from build123d import *

# Parameters (mm, degrees)
SKETCH1_R           = 2.032
BOSS_EXTRUDE1_DEPTH = 7.62
SKETCH3_W           = 2.54
SKETCH3_H           = 7.62
CUT_EXTRUDE1_DEPTH  = 55.88
FILLET2_R           = 4.064
SKETCH5_W           = 8.89
SKETCH5_H           = 7.62
SKETCH5_R           = 1.905
BOSS_EXTRUDE2_DEPTH = 5.08
FILLET3_R           = 1.27
FILLET4_R           = 0.0508


with BuildPart() as part:
    # Sketch1 → Boss-Extrude1 (new body)
    with BuildSketch(Plane.XY):
        Polygon((0, 0), (0, 12.7), (7.62, 12.7), (7.62, 5.08), (48.26, 5.08), (48.26, 12.7), (55.88, 12.7), (55.88, 0), align=None)
        with Locations((3.81, 8.89)):
            Circle(SKETCH1_R, mode=Mode.SUBTRACT)
        with Locations((52.07, 8.89)):
            Circle(SKETCH1_R, mode=Mode.SUBTRACT)
    extrude(amount=-BOSS_EXTRUDE1_DEPTH)

    # Sketch3 → Cut-Extrude1 (cut)
    with BuildSketch(Plane(origin=(55.88, 0, 0), x_dir=(0, 0, -1), z_dir=(1, 0, 0))):
        with Locations((3.81, 8.89)):
            Rectangle(SKETCH3_W, SKETCH3_H)
    extrude(amount=-CUT_EXTRUDE1_DEPTH, mode=Mode.SUBTRACT)

    # Fillet2
    # the kernel refuses this fillet: 4.064 mm, written as the material it takes off along each edge
    with BuildSketch(Plane(origin=(48.26, 12.7, 5.08), x_dir=(0, -1, 0), z_dir=(0, 0, -1)), Plane(origin=(48.26, 12.7, 10.16), x_dir=(0, -1, 0), z_dir=(0, 0, -1)), Plane(origin=(7.62, 12.7, 5.08), x_dir=(-1, 0, 0), z_dir=(0, 0, -1)), Plane(origin=(7.62, 12.7, 10.16), x_dir=(-1, 0, 0), z_dir=(0, 0, -1)), Plane(origin=(55.88, 12.7, 10.16), x_dir=(-1, 0, 0), z_dir=(0, 0, -1)), Plane(origin=(0, 12.7, 5.08), x_dir=(0, -1, 0), z_dir=(0, 0, -1)), Plane(origin=(0, 12.7, 10.16), x_dir=(0, -1, 0), z_dir=(0, 0, -1))) as fillet2_piece_1:
        with BuildLine():
            CenterArc((FILLET2_R, -FILLET2_R), FILLET2_R, 90, 90)
            Line((0, -FILLET2_R), (0, 0))
            Line((0, 0), (FILLET2_R, 0))
        make_face()
    extrude(amount=22.86, mode=Mode.SUBTRACT)
    with BuildSketch(Plane(origin=(55.88, 12.7, 5.08), x_dir=(0, -1, 0), z_dir=(0, 0, -1))) as fillet2_piece_2:
        with BuildLine():
            CenterArc((FILLET2_R, FILLET2_R), FILLET2_R, 180, 90)
            Line((0, FILLET2_R), (0, 0))
            Line((0, 0), (FILLET2_R, 0))
        make_face()
    extrude(amount=22.86, mode=Mode.SUBTRACT)

    # Sketch5 → Boss-Extrude2 (add)
    # profile 1 of 2: a face of its own
    with BuildSketch(Plane(origin=(0, 0, 0), x_dir=(1, 0, 0), z_dir=(0, 1, 0))):
        with Locations((-4.445, 3.81)):
            Rectangle(SKETCH5_W, SKETCH5_H)
        with Locations(Location((-5.08, 3.81, 0), (0, 0, 270))):
            Circle(SKETCH5_R, mode=Mode.SUBTRACT)
    # profile 2 of 2: a face of its own
    with BuildSketch(Plane(origin=(0, 0, 0), x_dir=(1, 0, 0), z_dir=(0, 1, 0))):
        with Locations((60.325, 3.81)):
            Rectangle(SKETCH5_W, SKETCH5_H)
        with Locations(Location((60.96, 3.81, 0), (0, 0, 270))):
            Circle(SKETCH5_R, mode=Mode.SUBTRACT)
    extrude(amount=BOSS_EXTRUDE2_DEPTH)

    # Fillet3
    fillet3_edges = [part.edges().sort_by_distance(p)[0] for p in [
        (0, 5.08, -1.27),
        (0, 5.08, -6.35),
        (55.88, 5.08, -6.35),
        (55.88, 5.08, -1.27),
        (7.62, 5.08, -6.35),
        (48.26, 5.08, -6.35),
        (48.26, 5.08, -1.27),
        (7.62, 5.08, -1.27),
    ]]
    fillet(fillet3_edges, radius=FILLET3_R)

    # Fillet4
    fillet4_edges = [part.edges().sort_by_distance(p)[0] for p in [
        (3.81, 5.08, -5.08),
        (3.81, 5.08, -2.54),
        (52.07, 5.08, -2.54),
        (52.07, 5.08, -5.08),
    ]]
    fillet(fillet4_edges, radius=FILLET4_R)


solid = part.part
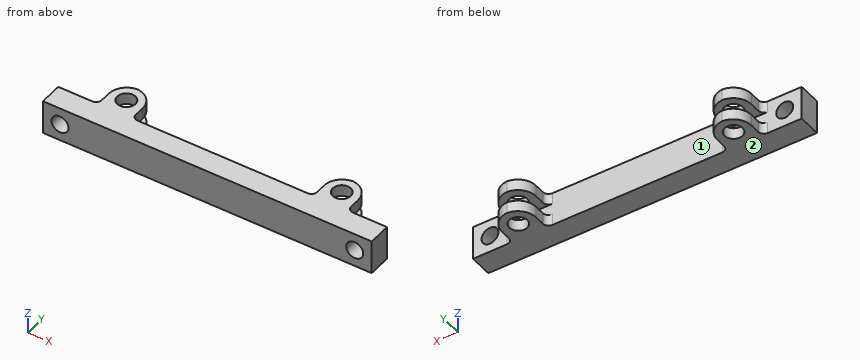
Geometry check sheet. Reference: the model listing, model coordinates, mm. Face numbers are marked on the shaded views. Round coordinates to 2 decimals unless told otherwise and drop trailing zeros. Write each loop counter-clockwise with the first axis right and the second up, starting at its lowest first coordinate (ties: lowest second). Pieces come first, ordered by that corner, then holes. Notation, with made-up numbers: (69, -13.5) - (95, -13.5) arc R25 ccw to (95, 22.5) - close; hole circle Ø8 at (-9, -1.75). An arc over 180 degrees is marked (long way). One line per item, written item: value.
1. Mould release check, pull along X, two halves, no side actions. Record for the marked faces 1 and 2: released by +X, released by -X, zero draft, split by the parting line, or undercut.
The answers:
face 1: undercut
face 2: zero draft
2. Cross-section at A-A on x = 60.96. Record the boundary of the cut face in (y, z) (3 decimals).
The answers:
outline: (0, -7.62) - (5.08, -7.62) - (5.08, -5.715) - (0, -5.715) - close; (0, -1.905) - (5.08, -1.905) - (5.08, 0) - (0, 0) - close
3. Depth check by flat-ended pin: pin 1 Ø4 at (x, y) = (2.5, 10) entering from +Z; pin 2 Ø0.7 at (y, z) = (7, -1.5) entering from +X; pin 3 Ø0.7 at (y, z) = (7, -1.5) entering from -X; pin 4 Ø2.5 at (x, z) = (12, -3.5) entering from +Y. Enter the tip coordinate at first touch or a pass-through.
The answers:
pin 1: stops at z = 0
pin 2: stops at x = 55.88
pin 3: stops at x = 0
pin 4: stops at y = 5.08
4. Cross-section at D-D on y = 10.25. Give the number of separate pieces and of enclosed holes in the cut face, and give its area (3 significant figures).
The answers:
separate pieces: 8
enclosed holes: 0
area: 39.9 mm^2
5. Cross-section at C-C on y = 4. Record the boundary of the cut face in (x, z) (3 decimals).
The answers:
outline: (-8.89, -7.62) - (64.77, -7.62) - (64.77, 0) - (-8.89, 0) - close; hole circle Ø3.81 at (-5.08, -3.81); hole circle Ø3.81 at (60.96, -3.81)
6. Cross-section at B-B on z = -1.25. Record the boundary of the cut face in (x, y).
The answers:
outline: (-8.89, 0) - (64.77, 0) - (64.77, 5.08) - (57.15, 5.08) arc R1.27 cw to (55.88, 6.35) - (55.88, 8.64) arc R4.06 ccw to (52.07, 12.69) arc R4.06 ccw to (48.26, 8.64) - (48.26, 6.35) arc R1.27 cw to (46.99, 5.08) - (8.89, 5.08) arc R1.27 cw to (7.62, 6.35) - (7.62, 8.64) arc R4.06 ccw to (3.81, 12.69) arc R4.06 ccw to (0, 8.64) - (0, 6.35) arc R1.27 cw to (-1.27, 5.08) - (-8.89, 5.08) - close; hole circle Ø4.06 at (3.81, 8.89); hole circle Ø4.06 at (52.07, 8.89)
7. Scan lines: L1, parallel to X at y = 3, z = -3.81 (3 decimals); L2, parallel to X at y = 10, z = -1.25; L3, parallel to Z at x = 2, y = 7. Record each from-to range of solid material in increasing order.
The answers:
L1: x = -8.89 to -6.985, -3.175 to 59.055, 62.865 to 64.77
L2: x = 0.24 to 2.11, 5.51 to 7.38, 48.5 to 50.37, 53.77 to 55.64
L3: z = -7.62 to -5.08, -2.54 to 0
